The drawing under review shows one solid part. Ordinate dimensions are in mm from its lowest x, y, z. Coordinates: 2 decimals unless noted, no trailing zeros. Order: outer loops, then holes, each group sorted by start corner. A loop starts at its lowest first (then second) coordinate and runs counter-clockwise, first axis right, second up. Notation, with made-up numbers: (6, 43) -> (50, 43) arc R20 cw to (50, 61) -> close; hole circle Ø7 at (6, 24). An arc over 180 degrees is marked (long way). Put each result on its own line as item: value.
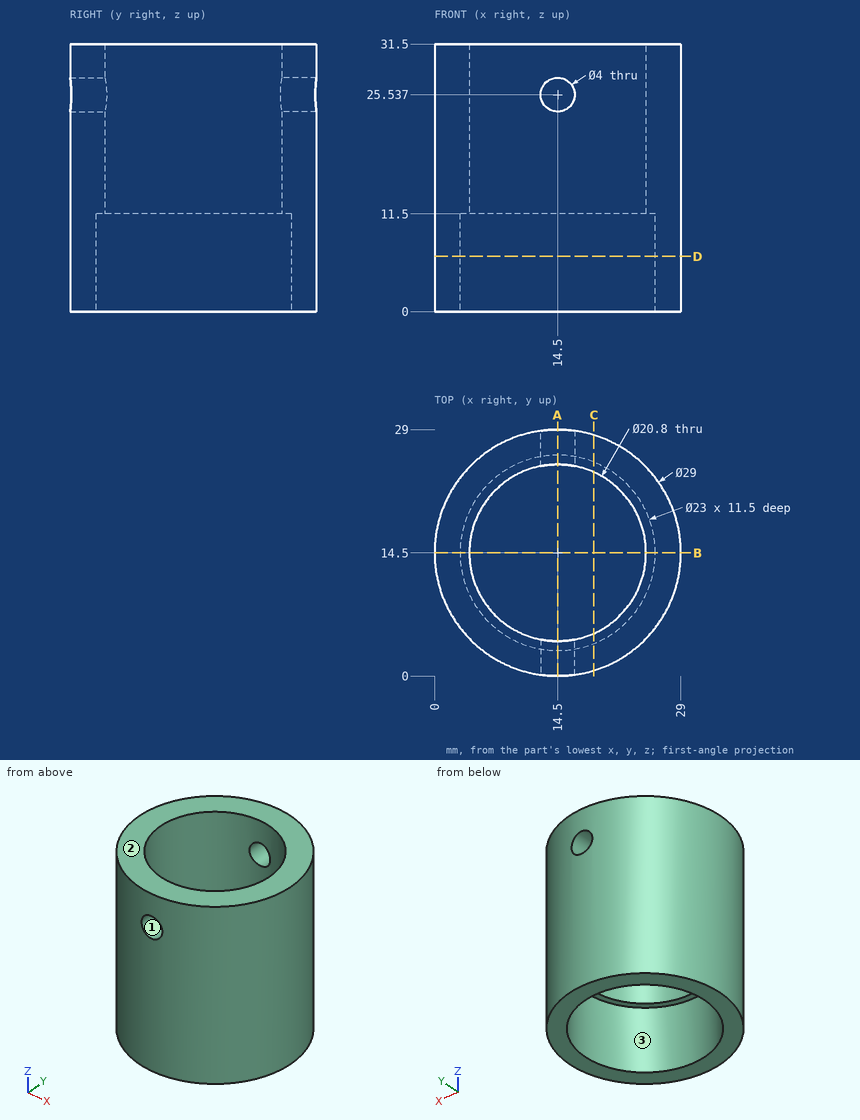
Item 1: For line 1 (Y direction, x = 14.5, z = 6.75); line 2 (Z direction, x = 14.5, y = 25.75); line 3 (Z direction, x = 14.5, y = 26.6), list the stretches that pass through material, from the lowest coordinate up. Write a range as from..to.
Answers below:
line 1: 0..3, 26..29
line 2: 11.5..23.54, 27.54..31.5
line 3: 0..23.54, 27.54..31.5
Item 2: Consider section B-B on y = 14.5. Write out the cut boundary in (x, z).
Answers below:
outline: (0, 0) -> (3, 0) -> (3, 11.5) -> (4.1, 11.5) -> (4.1, 31.5) -> (0, 31.5) -> close; (24.9, 11.5) -> (26, 11.5) -> (26, 0) -> (29, 0) -> (29, 31.5) -> (24.9, 31.5) -> close
Item 3: Mouldability with a two-part tool opening along Z and no side actions: class the marked faces 1, 2 and 3 as +Z half, -Z half, draft (parallel to the pull), parting line (faces both ways), or undercut.
Answers below:
face 1: undercut
face 2: +Z half
face 3: draft
Item 4: Consider section D-D on z = 6.5. Write out the cut boundary in (x, y).
Answers below:
outline: circle Ø29 at (14.5, 14.5); hole circle Ø23 at (14.5, 14.5)
Item 5: For pin 1 Ø10 at (x, z) = (20, 22) entering from +Y; pin 2 Ø1 at (x, z) = (26, 17) entering from -Y; pin 3 Ø2 at (x, z) = (16.5, 16.5) entering from -Y, all flat-tipped, find the tip position at first contact; note any pin that passes through.
Answers below:
pin 1: y = 28.99
pin 2: y = 5.05
pin 3: y = 0.03
Item 6: Consider section A-A on x = 14.5. Write out the cut boundary in (y, z), and give its area (3 significant figures).
Answers below:
outline: (0, 0) -> (3, 0) -> (3, 11.5) -> (4.1, 11.5) -> (4.1, 23.54) -> (0, 23.54) -> close; (0, 27.54) -> (4.1, 27.54) -> (4.1, 31.5) -> (0, 31.5) -> close; (24.9, 11.5) -> (26, 11.5) -> (26, 0) -> (29, 0) -> (29, 23.54) -> (24.9, 23.54) -> close; (24.9, 27.54) -> (29, 27.54) -> (29, 31.5) -> (24.9, 31.5) -> close
area: 200 mm^2
Item 7: Consider section C-C on x = 18.75. Write out the cut boundary in (y, z), and give its area (3 significant figures).
Answers below:
outline: (0.64, 0) -> (3.81, 0) -> (3.81, 11.5) -> (5.01, 11.5) -> (5.01, 31.5) -> (0.64, 31.5) -> close; (23.99, 11.5) -> (25.19, 11.5) -> (25.19, 0) -> (28.36, 0) -> (28.36, 31.5) -> (23.99, 31.5) -> close
area: 248 mm^2
